Read the model definition and answer for the solid it produces. Units are mm, in the model's axes. Coordinates: 2 decimals unless noted, no trailing zeros. Write each loop counter-clockwise with the first axis right and the second up, starting at its lowest first coordinate (ties: lowest second). Pieces come first, ordered by that corner, then holes. Notation, with made-up numbers: (-7.75, 37.5) -> (-1.75, 37.5) arc R24 ccw to (-1.75, 70.5) -> close; hole circle Ø1 at (11, 66). An arc over 180 degrees is marked (long way). Answer in a Markdown table with one row per item. Add a question column.
Item 1: Straight lines are drawn through the part: line 1 (Y direction, x = 20, z = 0.85); line 2 (Z direction, x = 4, y = 2); line 3 (X direction, y = 0.75, z = 31). For each, find the intervals that lie inside material, in ascending order. Write a range as from..to.
Item 2: Section A-A on x = 20 is taken. Write down the section's boundary in (y, z), then the cut area to 3 significant figures.
Item 3: Given pin 1 Ø6 at (x, y) = (48.5, -2.5) entering from +Z; pin 2 Ø5 at (x, y) = (10.5, 1.5) entering from +Z; pin 3 Ø6 at (y, z) = (1, 28) entering from +X, each flat-ended and moving along its own axis, determine where each tip first touches the part or whether it passes through.
Item 4: Section B-B on y = 0 is taken. Write down the section's boundary in (x, z).
```python
from build123d import *

# Parameters (mm, degrees)
SKETCH1_R           = 2.5
BOSS_EXTRUDE1_DEPTH = 2
SKETCH2_R           = 2.5
BOSS_EXTRUDE2_DEPTH = 10
BOSS_EXTRUDE3_REACH = 123.214
SKETCH4_R           = 2.5
BOSS_EXTRUDE4_REACH = 164.331
SKETCH5_R           = 2.5


with BuildPart() as part:
    # Sketch1 → Boss-Extrude1 (new body)
    with BuildSketch(Plane.XY):
        with BuildLine():
            Line((0, 5), (40, 5))
            ThreePointArc((40, 5), (45, 0), (40, -5))
            Line((40, -5), (0, -5))
            ThreePointArc((0, -5), (-5, 0), (0, 5))
        make_face()
        with Locations((20, 0)):
            Circle(SKETCH1_R, mode=Mode.SUBTRACT)
    extrude(amount=BOSS_EXTRUDE1_DEPTH)

    # Sketch2 → Boss-Extrude2 (add)
    with BuildSketch(Plane.XY.offset(2)):
        Circle(SKETCH2_R)
        with Locations((40, 0)):
            Circle(SKETCH2_R)
    extrude(amount=BOSS_EXTRUDE2_DEPTH)

    # Boss-Extrude3: up to this plane
    boss_extrude3_end = Plane(origin=(0, 0, 12), z_dir=(0, 0, 1))
    # Sketch4 → Boss-Extrude3 (add, up to the surface)
    with BuildSketch(Plane(origin=(-51.423008775, 0, 73.28355545), x_dir=(0.7660444431189768, 0, 0.6427876096865409), z_dir=(-0.6427876096865408, 0, 0.7660444431189767)), mode=Mode.PRIVATE) as boss_extrude3_sk1:
        Circle(SKETCH4_R)
    boss_extrude3_tool1 = split(extrude(boss_extrude3_sk1.sketch, amount=-BOSS_EXTRUDE3_REACH, mode=Mode.PRIVATE), bisect_by=boss_extrude3_end, keep=Keep.BOTH, mode=Mode.PRIVATE)
    add(boss_extrude3_tool1.solids().sort_by_distance((-51.423009, 0, 73.283555))[0])

    # Boss-Extrude4: up to this plane
    boss_extrude4_end = Plane(origin=(40, 0, 12), z_dir=(0, 0, 1))
    # Sketch5 → Boss-Extrude4 (add, up to the surface)
    with BuildSketch(Plane(origin=(91.423008775, 0, 73.28355545), x_dir=(0.7660444431189772, 0, -0.6427876096865404), z_dir=(0.6427876096865403, 0, 0.7660444431189771)), mode=Mode.PRIVATE) as boss_extrude4_sk1:
        Circle(SKETCH5_R)
    boss_extrude4_tool1 = split(extrude(boss_extrude4_sk1.sketch, amount=-BOSS_EXTRUDE4_REACH, mode=Mode.PRIVATE), bisect_by=boss_extrude4_end, keep=Keep.BOTH, mode=Mode.PRIVATE)
    add(boss_extrude4_tool1.solids().sort_by_distance((91.423009, 0, 73.283555))[0])


solid = part.part
```
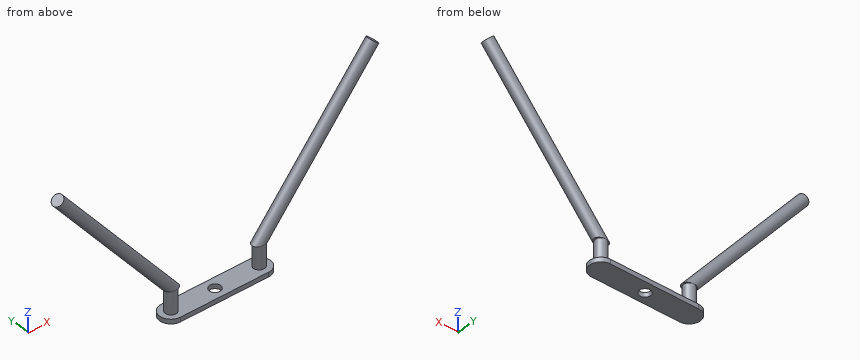
Results below:
| question | item | result |
|---|---|---|
| 1 | line 1 | y = -5..-2.5, 2.5..5 |
| 1 | line 2 | z = 0..2 |
| 1 | line 3 | x = -19.06..-12.83, 52.83..59.06 |
| 2 | outline | (-5, 0) -> (-2.5, 0) -> (-2.5, 2) -> (-5, 2) -> close; (2.5, 0) -> (5, 0) -> (5, 2) -> (2.5, 2) -> close |
| 2 | area | 10.0 mm2 |
| 3 | pin 1 | stops at z = 28.79 |
| 3 | pin 2 | stops at z = 2 |
| 3 | pin 3 | stops at x = 59.11 |
| 4 | outline | (-53.34, 71.68) -> (-3.26, 12) -> (-2.5, 12) -> (-2.5, 2) -> (-5, 2) -> (-5, 0) -> (17.5, 0) -> (17.5, 2) -> (2.5, 2) -> (2.5, 12) -> (3.26, 12) -> (-49.51, 74.89) -> close; (22.5, 0) -> (45, 0) -> (45, 2) -> (42.5, 2) -> (42.5, 12) -> (43.26, 12) -> (93.34, 71.68) -> (89.51, 74.89) -> (36.74, 12) -> (37.5, 12) -> (37.5, 2) -> (22.5, 2) -> close |
